CAD build for the part. Positions are in the model's coordinates, mm. A direction names the side the tool comes from. Round coordinates to 2 decimals unless told otherwise and drop trailing zeros. Loops run counter-clockwise (first coordinate to the right, second up) from the corner with the lowest first, then second, coordinate; pieces in that order, holes last. Notation, with made-up numbers: (77, -28) - (107, -28) arc R23 ccw to (107, -8) - close; hole circle Ø11 at (53.25, -6.5). An arc over 180 degrees is marked (long way). Use one line per item in the form item = value.
from build123d import *

# Parameters (mm, degrees)
SKETCH1_W           = 614.68
SKETCH1_H           = 30.48
BOSS_EXTRUDE1_DEPTH = 15.24
SKETCH2_W           = 15.24
SKETCH2_H           = 2.54
CUT_EXTRUDE1_DEPTH  = 15.24
SKETCH3_W           = 15.24
SKETCH3_H           = 25.4
CUT_EXTRUDE2_DEPTH  = 2.54
SKETCH4_R           = 5.08
CUT_EXTRUDE3_DEPTH  = 17.78
SKETCH5_W           = 50.8
SKETCH5_H           = 15.24
CUT_EXTRUDE4_DEPTH  = 7.62
SKETCH6_R           = 5.08
CUT_EXTRUDE5_DEPTH  = 12.7
SKETCH7_R           = 5.08
CUT_EXTRUDE6_DEPTH  = 17.78


with BuildPart() as part:
    # Sketch1 → Boss-Extrude1 (new body)
    with BuildSketch(Plane(origin=(0, 0, 0), x_dir=(1, 0, 0), z_dir=(0, 1, 0))):
        Rectangle(SKETCH1_W, SKETCH1_H)
    extrude(amount=BOSS_EXTRUDE1_DEPTH)

    # Sketch2 → Cut-Extrude1 (cut)
    with BuildSketch(Plane(origin=(0, 15.24, 0), x_dir=(1, 0, 0), z_dir=(0, 1, 0))):
        with Locations((-299.72, 13.97)):
            Rectangle(SKETCH2_W, SKETCH2_H)
        with Locations((-299.72, -13.97)):
            Rectangle(SKETCH2_W, SKETCH2_H)
        with Locations((299.72, 13.97)):
            Rectangle(SKETCH2_W, SKETCH2_H)
        with Locations((299.72, -13.97)):
            Rectangle(SKETCH2_W, SKETCH2_H)
    extrude(amount=-CUT_EXTRUDE1_DEPTH, mode=Mode.SUBTRACT)

    # Sketch3 → Cut-Extrude2 (cut)
    with BuildSketch(Plane.XZ):
        with Locations((299.72, 0)):
            Rectangle(SKETCH3_W, SKETCH3_H)
        with Locations((-299.72, 0)):
            Rectangle(SKETCH3_W, SKETCH3_H)
    extrude(amount=-CUT_EXTRUDE2_DEPTH, mode=Mode.SUBTRACT)

    # Sketch4 → Cut-Extrude3 (cut)
    with BuildSketch(Plane(origin=(0, 15.24, 0), x_dir=(1, 0, 0), z_dir=(0, 1, 0))):
        with Locations(Location((-299.72, 0, 0), (0, 0, 270))):
            Circle(SKETCH4_R)
        with Locations(Location((299.72, 0, 0), (0, 0, 270))):
            Circle(SKETCH4_R)
    extrude(amount=-CUT_EXTRUDE3_DEPTH, mode=Mode.SUBTRACT)

    # Sketch5 → Cut-Extrude4 (cut)
    with BuildSketch(Plane(origin=(0, 15.24, 0), x_dir=(1, 0, 0), z_dir=(0, 1, 0))):
        with Locations((0, -7.62)):
            Rectangle(SKETCH5_W, SKETCH5_H)
    extrude(amount=-CUT_EXTRUDE4_DEPTH, mode=Mode.SUBTRACT)

    # Sketch6 → Cut-Extrude5 (cut)
    with BuildSketch(Plane(origin=(0, 7.62, 0), x_dir=(1, 0, 0), z_dir=(0, 1, 0))):
        with Locations(Location((0, -7.62, 0), (0, 0, 270))):
            Circle(SKETCH6_R)
    extrude(amount=-CUT_EXTRUDE5_DEPTH, mode=Mode.SUBTRACT)

    # Sketch7 → Cut-Extrude6 (cut)
    with BuildSketch(Plane(origin=(0, 15.24, 0), x_dir=(1, 0, 0), z_dir=(0, 1, 0))):
        with Locations(Location((-279.4, -7.62, 0), (0, 0, 270))):
            Circle(SKETCH7_R)
        with Locations(Location((-256.54, -7.62, 0), (0, 0, 270))):
            Circle(SKETCH7_R)
        with Locations(Location((-233.68, -7.62, 0), (0, 0, 270))):
            Circle(SKETCH7_R)
        with Locations(Location((-210.82, -7.62, 0), (0, 0, 270))):
            Circle(SKETCH7_R)
        with Locations(Location((279.4, -7.62, 0), (0, 0, 270))):
            Circle(SKETCH7_R)
        with Locations(Location((256.54, -7.62, 0), (0, 0, 270))):
            Circle(SKETCH7_R)
        with Locations(Location((233.68, -7.62, 0), (0, 0, 270))):
            Circle(SKETCH7_R)
        with Locations(Location((210.82, -7.62, 0), (0, 0, 270))):
            Circle(SKETCH7_R)
    extrude(amount=-CUT_EXTRUDE6_DEPTH, mode=Mode.SUBTRACT)


solid = part.part
1) Tool access for faces 1 (the flat face through (-300, 9, 12.7)), 2 (the flat face through (299.6, 2.54, -5.5)), 3 (the flat face through (300, 9, 12.7)): list every direction of +Z, -Z, +X, -X, +Y, -Y with a clear straight run to the whole face (end or side of a thin tool).
Report:
face_1 = +Z, -X, +Y, -Y
face_2 = +Z, -Z, +X, -Y
face_3 = +Z, +X, +Y, -Y
2) Two-plate mould, pull along X, no slides. Class faces 4 (the flat face through (-300, 9, -12.7)), 5 (the flat face through (-307.34, 9, 0)), 6 (the cylindrical face through (-304.68, 8.98, -1.1)): +X half, -X half, draft (parallel to the pull), parting line (faces both ways), or undercut.
Report:
face_4 = draft
face_5 = -X half
face_6 = undercut
3) Drill centre lines: probe 1 along Z at (x, y) = (279.4, 6); probe 2 along Z at (x, y) = (278.5, 4.5); probe 3 along X at (y, z) = (1, -2). Where is each one in solid material? Low to high.
Report:
probe_1 = -15.24 to 2.54, 12.7 to 15.24
probe_2 = -15.24 to 2.62, 12.62 to 15.24
probe_3 = -292.1 to 292.1
4) Slice it at A-A (x = -279.4). Write the cut outline in (y, z), plus the area to 3 significant figures.
Report:
outline = (0, -15.24) - (15.24, -15.24) - (15.24, 2.54) - (0, 2.54) - close; (0, 12.7) - (15.24, 12.7) - (15.24, 15.24) - (0, 15.24) - close
area = 310 mm^2
5) Flat gauge pins, fed straight in: pin 1 (4.5 mm diameter, centred on x = 11.5, z = 4.5, fed in from +Y); pin 2 (13 mm diameter, centred on x = 299.72, z = 0, fed in from -Y); pin 3 (2.5 mm diameter, centred on x = 10, y = 11, fed in from +Z). Where does each tip first touch, or does it go through?
Report:
pin_1 = 7.62
pin_2 = 2.54
pin_3 = 0
